Geometry: final body of the model. Coordinates: model frame, mm. A direction names the side the tool comes from. Coordinates: 2 decimals unless noted, no trailing zeros. One line per item, written item: value. Start each with the question number.
Item 1: Contact query for flat-ended pins moving along their axis: pin 1 Ø11 at (x, y) = (43, -6.5) entering from +Z; pin 2 Ø5 at (y, z) = (-19.5, 13.5) entering from +X; pin 3 Ø9 at (x, y) = (48.5, -8.5) entering from -Z. Output: stop coordinate, or through.
Item 2: Mould query, pull axis X, two halves, no side actions, for faces 5 (the flat face through (46, 41, 38)), 6 (the flat face through (-39.5, 1, 38)), 7 (the flat face through (1, -41, 38)), 8 (the cylindrical face through (-38.07, -39.5, 37.31)). Classes: +X half, -X half, draft (parallel to the pull), parting line (faces both ways), or undercut.
Item 3: Ray query, probe 1 along Y at (x, z) = (4.5, 53); probe 2 along X at (y, z) = (-3, 25.5); probe 3 along Y at (x, z) = (46.5, 59). Return the intervals inside material, ascending. Write a range as from..to.
Item 4: Set-up query: faces 1 (the flat face through (46, 1, 1)), 2 (the flat face through (46, -41, 37)), 3 (the cylindrical face through (-38, 39.57, 37.31)), 4 (the cylindrical face through (45, -38, 3)). Return all of +Z, -Z, +X, -X, +Y, -Y with unobstructed straight access to the full face (end or side cutting, diameter ignored); none if empty.
from build123d import *

# Parameters (mm, degrees)
F0_W     = 81
F0_H     = 84
F1_DEPTH = 70
F3_DEPTH = 69
F5_DEPTH = 2
F7_DEPTH = 14
F8_R     = 5
F9_R     = 0.49999


# Not quite as in the source:
# - a fillet or chamfer is up to 0.001 mm smaller than in the source, because OpenCascade refuses the exact size


with BuildPart() as f1:
    # F0 (on Top) → F1 (new body)
    with BuildSketch(Plane.XY):
        Rectangle(F0_W, F0_H)
    extrude(amount=F1_DEPTH)

    # F2 (on face) → F3 (cut)
    with BuildSketch(Plane.XY.offset(70)):
        Polygon((38.5, 41), (-39.5, 41), (-39.5, 20.586034283), (-39.5, -41), (38.5, -41), (38.5, -37.5405208561), align=None)
    extrude(amount=-F3_DEPTH, mode=Mode.SUBTRACT)

    # F4 (on face) → F5 (cut)
    with BuildSketch(Plane.YZ.offset(40.5)):
        Polygon((40, 2), (40, 70), (-40, 70), (-40, 42.2970801592), (-40, 2), align=None)
    extrude(amount=-F5_DEPTH, mode=Mode.SUBTRACT)

    # F6 (on face) → F7 (join)
    with BuildSketch(Plane(origin=(38.5, 0, 0), x_dir=(0, -1, 0), z_dir=(-1, 0, 0))):
        Polygon((41, 1), (41, 70), (40, 70), (40, 2), (-40, 2), (-40, 70), (-41, 70), (-41, 1), align=None)
    extrude(amount=-F7_DEPTH)

    # F8
    f8_edges = [f1.edges().sort_by_distance(p)[0] for p in [
        (-0.5, 41, 1),
        (-39.5, 0, 1),
        (-0.5, -41, 1),
        (0, 42, 0),
        (-40.5, 0, 0),
        (0, -42, 0),
        (-40.5, -42, 35),
        (-40.5, 42, 35),
        (-39.5, 41, 35.5),
        (-39.5, -41, 35.5),
        (46.5, 41, 1),
        (46.5, -41, 1),
        (45.5, -40, 2),
        (45.5, 40, 2),
    ]]
    fillet(f8_edges, radius=F8_R)

    # F9 (radius 0.5 in the source; OpenCascade refuses exactly that, so slightly less here)
    f9_edges = [f1.edges().sort_by_distance(p)[0] for p in [
        (2.5, 42, 70),
        (-39.035534, 40.535534, 70),
        (40.5, 41.5, 70),
        (-40.5, 0, 70),
        (46.5, 41, 70),
        (-39.035534, -40.535534, 70),
        (52.5, 40.5, 70),
        (2.5, -42, 70),
        (45.5, 40, 70),
        (40.5, -41.5, 70),
        (38.5, 40.5, 70),
        (46.5, -41, 70),
        (2, 41, 70),
        (52.5, -40.5, 70),
        (-38.035534, 39.535534, 70),
        (45.5, -40, 70),
        (-39.5, 0, 70),
        (38.5, -40.5, 70),
        (-38.035534, -39.535534, 70),
        (2, -41, 70),
        (52.5, -41, 38),
        (52.5, -39.535534, 2.464466),
        (52.5, 0, 1),
        (52.5, -40, 38.5),
        (52.5, 39.535534, 2.464466),
        (52.5, -38.535534, 3.464466),
        (52.5, 41, 38),
        (52.5, 0, 2),
        (52.5, 38.535534, 3.464466),
        (52.5, 40, 38.5),
    ]]
    fillet(f9_edges, radius=F9_R)


solid = f1.part
Reply:
1. pin 1: stops at z = 2
1. pin 2: stops at x = -39.5
1. pin 3: stops at z = 1
2. face 5: draft
2. face 6: +X half
2. face 7: undercut
2. face 8: undercut
3. probe 1: y = -42..-41, 41..42
3. probe 2: x = -40.5..-39.5
3. probe 3: y = -41..-40, 40..41
4. face 1: -Z, +X, +Y, -Y
4. face 2: +Z, -Z, +X, -Y
4. face 3: +Z
4. face 4: +Z, +X
